from build123d import *

# Parameters (mm, degrees)
BOSS_EXTRUDE1_DEPTH = 68.58
SKETCH3_R           = 19.05
SKETCH3_R_2         = 6.35
BOSS_EXTRUDE2_DEPTH = 6.35
SKETCH3_3_R         = 6.35
BOSS_EXTRUDE3_DEPTH = 19.05


with BuildPart() as part:
    # Sketch1 → Boss-Extrude1 (new body)
    with BuildSketch(Plane.XY):
        with BuildLine():
            Line((-49.186888497, 12.7), (-36.486888497, 12.7))
            Line((-36.486888497, 12.7), (-36.486888497, -12.7))
            Line((-36.486888497, -12.7), (-49.186888497, -12.7))
            ThreePointArc((-49.186888497, -12.7), (0, -50.8), (49.186888497, -12.7))
            Line((49.186888497, -12.7), (36.486888497, -12.7))
            Line((36.486888497, -12.7), (36.486888497, 12.7))
            Line((36.486888497, 12.7), (49.186888497, 12.7))
            ThreePointArc((49.186888497, 12.7), (0, 50.8), (-49.186888497, 12.7))
        make_face()
    extrude(amount=BOSS_EXTRUDE1_DEPTH)

    # Sketch3 → Boss-Extrude2 (add, symmetric)
    with BuildSketch(Plane(origin=(0, 0, 0), x_dir=(0, 0, -1), z_dir=(1, 0, 0))):
        with Locations((58.42, 0)):
            Circle(SKETCH3_R)
        with Locations((58.42, 0)):
            Circle(SKETCH3_R_2, mode=Mode.SUBTRACT)
        with BuildLine():
            Line((44.220968343, 12.7), (0, 12.7))
            Line((0, 12.7), (0, -12.7))
            Line((0, -12.7), (44.220968343, -12.7))
            ThreePointArc((44.220968343, -12.7), (39.37, 0), (44.220968343, 12.7))
        make_face()
    extrude(amount=BOSS_EXTRUDE2_DEPTH, both=True)

    # Sketch3_3 → Boss-Extrude3 (add, symmetric)
    with BuildSketch(Plane(origin=(0, 0, 0), x_dir=(0, 0, -1), z_dir=(1, 0, 0))):
        with Locations((58.42, 0)):
            Circle(SKETCH3_3_R)
    extrude(amount=BOSS_EXTRUDE3_DEPTH, both=True)


solid = part.part
For this review, take the finished solid that the model builds, in its own axes (mm). A direction names the side the tool comes from. Coordinates: 2 decimals unless noted, no trailing zeros. Write each loop counter-clockwise with the first axis right and the second up, starting at its lowest first coordinate (ties: lowest second). Pieces come first, ordered by that corner, then holes. Notation, with made-up numbers: (36.25, 28.25) -> (92.25, 28.25) arc R11 ccw to (92.25, 46.25) -> close; hole circle Ø6 at (-1, 34). An arc over 180 degrees is marked (long way). Write each question's results on one line, items separated by ' | '. Start each with the question number.
1) The part is to be moulded in two halves that separate along Y. For faces 1 (the face through (43, -12.7, 34)), 2 (the face through (12.789, 1.907, -64.477)), 3 (the face through (-1, 1, 68.58)), say which applies: +Y half, -Y half, draft (parallel to the pull), parting line (faces both ways), or undercut.
2) Insertion check: pin 1 (4 mm diameter, centred on y = 2, z = -57, fed in from -X); pin 2 (7.5 mm diameter, centred on y = 1.5, z = 29.5, fed in from -X); pin 3 (6 mm diameter, centred on x = 9, z = -8.5, fed in from +Y). Each pin has a flat end and moves straight along its axis. Give the tip position at first contact, or say it passes through.
3) Consider section B-B (x = 8). Write out the cut boundary in (y, z).
4) Wall thickness on L1, parallel to X at y = -5, z = 3; L2, parallel to Z at x = 37.5, y = -31; L3, parallel to X at y = 16, z = -66.5: over which ranges is each line inside the solid? List them lowest first. Write a range as [from, to].
5) For faces 4 (the face through (43, 12.7, 34)), 5 (the face through (0, 12.7, -22)), 6 (the face through (6.35, 0, -38)), 7 (the face through (-43, 12.7, 34)), 8 (the face through (19.05, 0, -58)), list the 3-axis set-ups (+Z, -Z, +X, -X, +Y, -Y) from which the entire face can be reached by the end or side of a thin tool; tool diameter is ignored.
6) Consider section C-C (y = 0). Write out the cut boundary in (x, z), plus the area to 3 significant figures.
7) Consider section D-D (z = -58.42). Write out the cut boundary in (x, y).
8) Consider section A-A (z = 26.5). Write out the cut boundary in (x, y).
Geometry says:
1) face 1: undercut | face 2: parting line | face 3: draft
2) pin 1: x = -19.05 | pin 2: x = -36.49 | pin 3: y = 12.7
3) outline: (-50.17, 0) -> (50.17, 0) -> (50.17, 68.58) -> (-50.17, 68.58) -> close; circle Ø12.7 at (0, -58.42)
4) L1: [-36.49, 36.49] | L2: [0, 68.58] | L3: [-6.35, 6.35]
5) face 4: +Z, -Z, +X | face 5: +X, -X, +Y | face 6: +X | face 7: +Z, -Z, -X | face 8: -Z, +X, +Y, -Y
6) outline: (-36.49, 0) -> (-6.35, 0) -> (-6.35, -52.07) -> (-19.05, -52.07) -> (-19.05, -64.77) -> (-6.35, -64.77) -> (-6.35, -77.47) -> (6.35, -77.47) -> (6.35, -64.77) -> (19.05, -64.77) -> (19.05, -52.07) -> (6.35, -52.07) -> (6.35, 0) -> (36.49, 0) -> (36.49, 68.58) -> (-36.49, 68.58) -> close | area: 6,310 mm^2
7) outline: (-19.05, -6.35) -> (-6.35, -6.35) -> (-6.35, -19.05) -> (6.35, -19.05) -> (6.35, -6.35) -> (19.05, -6.35) -> (19.05, 6.35) -> (6.35, 6.35) -> (6.35, 19.05) -> (-6.35, 19.05) -> (-6.35, 6.35) -> (-19.05, 6.35) -> close
8) outline: (-49.19, -12.7) arc R50.8 ccw to (49.19, -12.7) -> (36.49, -12.7) -> (36.49, 12.7) -> (49.19, 12.7) arc R50.8 ccw to (-49.19, 12.7) -> (-36.49, 12.7) -> (-36.49, -12.7) -> close
